```python
from build123d import *

# Parameters (mm, degrees)
F0_W      = 94.672728
F0_H      = 71.350906
F1_DEPTH  = 12.7
F3_DEPTH  = 12.701
F4_R      = 41.183466
F5_DEPTH  = 50.8
F6_R      = 32.333479
F7_DEPTH  = 50.801
F8_W      = 47.867391
F8_H      = 10.548822
F9_DEPTH  = 38.1
F11_DEPTH = 46.481614


with BuildPart() as f1:
    # F0 (on Top) → F1 (new body)
    with BuildSketch(Plane.XY):
        with Locations((-9.467272, -1.847273)):
            Rectangle(F0_W, F0_H)
    extrude(amount=F1_DEPTH)

    # F2 (on face) → F3 (cut, through all)
    with BuildSketch(Plane.XY.offset(12.7)):
        with BuildLine():
            Line((37.869092, -37.522726), (37.869092, 33.82818))
            ThreePointArc((37.869092, 33.82818), (16.340406, -1.847273), (37.869092, -37.522726))
        make_face()
    extrude(amount=-F3_DEPTH, mode=Mode.SUBTRACT)

    # F4 (on Top) → F5 (join)
    with BuildSketch(Plane.XY):
        with Locations((50.53845, -1.962727)):
            Circle(F4_R)
    extrude(amount=F5_DEPTH)

    # F6 (on face) → F7 (cut, through all)
    with BuildSketch(Plane.XY.offset(50.8)):
        with Locations((50.53845, -1.962727)):
            Circle(F6_R)
    extrude(amount=-F7_DEPTH, mode=Mode.SUBTRACT)

    # F8 (on face) → F9 (join)
    with BuildSketch(Plane.XY.offset(12.7)):
        with Locations((-14.242494, -1.985464)):
            Rectangle(F8_W, F8_H)
    extrude(amount=F9_DEPTH)

    # F10 (on face) → F11 (cut, through all)
    with BuildSketch(Plane.XZ.offset(7.259875)):
        Polygon((-38.17619, 12.7), (9.691201, 50.8), (-38.17619, 50.8), align=None)
    extrude(amount=-F11_DEPTH, mode=Mode.SUBTRACT)


solid = f1.part
```
The model under review builds one solid part; all positions refer to its coordinate system, in mm. A direction names the side the tool comes from. Give positions to 0.01 mm unless a question says otherwise; leave off trailing zeros. Order: outer loops, then holes, each group sorted by start corner. A loop starts at its lowest first (then second) coordinate and runs counter-clockwise, first axis right, second up. Notation, with made-up numbers: (80, -21) - (88, -21) arc R30 ccw to (88, 14) - close; hole circle Ø2 at (39.25, 82). An arc over 180 degrees is marked (long way). Use CSV: the item, a comma, the result in double quotes. Start each with the question number.
Q1. We need section C-C, the plane z = 47. Write out the cut boundary in (x, y), and give its area (3 significant figures).
Q2. To check wall thickness, follow line 1 along Y through (x, z) = (-3.5, 19.5); line 2 along Y through (x, z) = (65.5, 43); line 3 along Y through (x, z) = (39.5, 16). State the ranges of each line that lie inside material, in increasing order. Write a range as [from, to].
Q3. We need section A-A, the plane x = 51. Write out the cut boundary in (y, z).
Q4. Clearance check with flat-ended pins moving along their axes: pin 1 Ø1.5 at (y, z) = (14.5, 7) entering from +X; pin 2 Ø4 at (x, z) = (61.5, 16.5) entering from +Y; pin 3 Ø10 at (x, z) = (-16.5, 4.5) entering from +Y; pin 4 Ø3 at (x, y) = (57.5, 26.5) entering from +Z (3 decimals). State where each tip first meets the part, or that it passes through.
Q5. The part is to be moulded in two halves that separate along Y. For faces 1 (the flat face through (-56.804, -2, 6)), 2 (the flat face through (-14, 33.828, 6)), 3 (the cylindrical face through (80.406, -14.347, 25.756)), 4 (the flat face through (-14, -37.523, 6)), say which applies: +Y half, -Y half, draft (parallel to the pull), parting line (faces both ways), or undercut.
Q6. We need section B-B, the plane y = -16. Write out the cut boundary in (x, z).
Q7. Tool access review of faces 5 (the flat face through (-14.58, -2.06, 31.48)), 6 (the flat face through (-24, 7, 12.7)), 7 (the flat face through (-9, -7.26, 27)), 8 (the flat face through (0, -1, 0)), 9 (the flat face through (-9, 3.289, 23)): name each direction out of +Z, -Z, +X, -X, +Y, -Y from which nothing blocks a thin tool from reaching the whole face with its end or side.
Q8. We need section D-D, the plane x = -3. Write out the cut boundary in (y, z), and give its area (3 significant figures).
Outcome:
1,outline,"(4.92, -7.26) - (9.69, -7.26) - (9.69, -7.21) arc R41.18 ccw (long way) to (9.69, 3.29) - (4.92, 3.29) - close; hole circle Ø64.67 at (50.54, -1.96)"
1,area,"2,090 mm^2"
2,line 1,"y = [-7.26, 3.29]"
2,line 2,"y = [-40.33, -30.63], [26.7, 36.41]"
2,line 3,"y = [-41.64, -32.35], [28.43, 37.71]"
3,outline,"(-43.14, 0) - (-34.29, 0) - (-34.29, 50.8) - (-43.14, 50.8) - close; (30.37, 0) - (39.22, 0) - (39.22, 50.8) - (30.37, 50.8) - close"
4,pin 1,"stops at x = 88.61"
4,pin 2,"stops at y = 38.23"
4,pin 3,"stops at y = 33.83"
4,pin 4,"passes through"
5,face 1,"draft"
5,face 2,"+Y half"
5,face 3,"undercut"
5,face 4,"-Y half"
6,outline,"(-56.8, 0) - (21.41, 0) - (21.41, 50.8) - (11.82, 50.8) - (11.82, 12.7) - (-56.8, 12.7) - close; (79.67, 0) - (89.26, 0) - (89.26, 50.8) - (79.67, 50.8) - close"
7,face 5,"+Z, -X, +Y, -Y"
7,face 6,"+Z, -X"
7,face 7,"+Z, -X, -Y"
7,face 8,"-Z, +X, -X, +Y, -Y"
7,face 9,"+Z, -X, +Y"
8,outline,"(-37.52, 0) - (33.83, 0) - (33.83, 12.7) - (3.29, 12.7) - (3.29, 40.7) - (-7.26, 40.7) - (-7.26, 12.7) - (-37.52, 12.7) - close"
8,area,"1,200 mm^2"
